Read the model definition and answer for the solid it produces. Units are mm, in the model's axes. A direction names the side the tool comes from. Coordinates: 2 decimals unless noted, no trailing zeros. Loops run counter-clockwise (first coordinate to the right, second up) from the corner with the lowest first, then second, coordinate; pieces in that order, holes last.
Q1. Section A-A (x = -20.5) is taken. Give the vertices of the cut face in (y, z), then the cut area to 3 significant figures.
Q2. Section D-D (y = -7) is taken. Give the vertices of the cut face in (x, z).
Q3. Section C-C (z = 2) is taken. Give the vertices of the cut face in (x, y).
Q4. The mould has two halves that part along X. Classify faces 1 (the face through (-19, -17.562, 3)), 2 (the face through (-22, -6, 3.9)), 3 (the face through (-18.32, -6.29, 1.92)), 4 (the face through (-8.367, -8, 2)): pulls with the +X half, pulls with the -X half, needs draft (parallel to the pull), parting line crosses it, or undercut.
Q5. Which of the six approach directions +Z, -Z, +X, -X, +Y, -Y give full straight-line access (tool end or side, diameter ignored) to faces 5 (the face through (-29.367, -8, 5)), 6 (the face through (-19, -7, 5))?
Q6. Straight lines are drawn through the part: line 1 (Z direction, x = -28, y = -4.5); line 2 (Z direction, x = -22, y = -4.25); line 3 (X direction, y = -13.75, z = 7.5). For each, find the intervals that lie inside material, in ascending order.
Q7. Section B-B (y = -4.75) is taken. Give the vertices of the cut face in (x, z), then the cut area to 3 significant figures.
Q8. Flat-ended cylindrical pins translate along their axes: P1, Ø1.5, axis at y = -3.5, z = 7.5, coming from the +X side; P2, Ø1.8, axis at x = -21.55, y = -7.63, coming from the -Z side; P3, Ø1.5, axis at x = -14.5, y = -5, coming from the +Z side; P4, Ø3.5, axis at x = -20.5, y = -6, coming from the -Z side. Find the tip coordinate at first contact, or state that the pin passes through.
from build123d import *

# Parameters (mm, degrees)
F0_W           = 1
F0_H           = 20
F1_DEPTH       = 10
F0_W_2         = 20
F2_DEPTH       = 5
F4_D           = 3
F4_CBORE_D     = 7
F4_CBORE_DEPTH = 3.9


with BuildPart() as f1:
    # F0 (on Top) → F1 (new body)
    with BuildSketch(Plane.XY):
        with Locations((-28.8674156551, -7.5615978579)):
            Rectangle(F0_W, F0_H)
    extrude(amount=F1_DEPTH)

    # F0 (on Top) → F2 (join)
    with BuildSketch(Plane.XY):
        with Locations((-18.3674156551, -7.5615978579)):
            Rectangle(F0_W_2, F0_H)
        with Locations((-28.8674156551, -7.5615978579)):
            Rectangle(F0_W, F0_H)
    extrude(amount=F2_DEPTH)

    # F4 (through all)
    with Locations(Plane(origin=(0, 0, 0), x_dir=(1, 0, 0), z_dir=(0, 0, -1))):
        with Locations((-21.5535256551, 7.6278164051)):
            CounterBoreHole(F4_D / 2, F4_CBORE_D / 2, F4_CBORE_DEPTH)


solid = f1.part
Numbers:
1. outline: (-17.56, 0) - (-10.97, 0) - (-10.97, 3.9) - (-8.7, 3.9) - (-8.7, 5) - (-17.56, 5) - close; (-6.56, 3.9) - (-4.29, 3.9) - (-4.29, 0) - (2.44, 0) - (2.44, 5) - (-6.56, 5) - close
1. area: 71.6 mm2
2. outline: (-29.37, 0) - (-25, 0) - (-25, 3.9) - (-22.92, 3.9) - (-22.92, 5) - (-28.37, 5) - (-28.37, 10) - (-29.37, 10) - close; (-20.19, 3.9) - (-18.11, 3.9) - (-18.11, 0) - (-8.37, 0) - (-8.37, 5) - (-20.19, 5) - close
3. outline: (-29.37, -17.56) - (-8.37, -17.56) - (-8.37, 2.44) - (-29.37, 2.44) - close; hole circle Ø7 at (-21.55, -7.63)
4. face 1: needs draft
4. face 2: undercut
4. face 3: undercut
4. face 4: pulls with the +X half
5. face 5: +Z, -Z, -X, +Y, -Y
5. face 6: +Z, +X, +Y, -Y
6. line 1: z = 0 to 5
6. line 2: z = 3.9 to 5
6. line 3: x = -29.37 to -28.37
7. outline: (-29.37, 0) - (-23.55, 0) - (-23.55, 3.9) - (-19.56, 3.9) - (-19.56, 0) - (-8.37, 0) - (-8.37, 5) - (-28.37, 5) - (-28.37, 10) - (-29.37, 10) - close
7. area: 94.5 mm2
8. P1: stops at x = -28.37
8. P2: passes through
8. P3: stops at z = 5
8. P4: stops at z = 0
